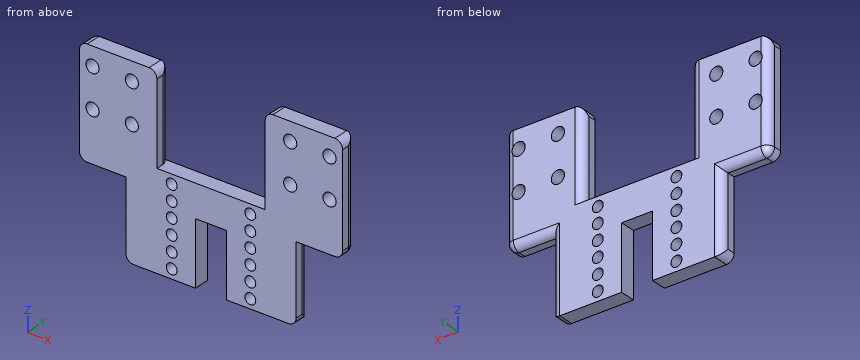
```python
from build123d import *

# Parameters (mm, degrees)
BOSS_EXTRUDE1_DEPTH  = 10
SKETCH2_R            = 4.25
CUT_EXTRUDE1_DEPTH   = 10
SKETCH3_R            = 3.5
CUT_EXTRUDE2_DEPTH   = 10
LPATTERN1_COUNT      = 2
LPATTERN1_PITCH      = 50.8
LPATTERN1_COUNT_DIR2 = 6
LPATTERN1_PITCH_DIR2 = 10
SKETCH4_W            = 30
SKETCH4_H            = 50
CUT_EXTRUDE3_DEPTH   = 10
FILLET1_R            = 5
SKETCH5_W            = 20
SKETCH5_H            = 41
CUT_EXTRUDE4_DEPTH   = 10


with BuildPart() as part:
    # Sketch1 → Boss-Extrude1 (new body)
    with BuildSketch(Plane(origin=(0, 0, 0), x_dir=(1, 0, 0), z_dir=(0, 1, 0))):
        Polygon((0, 0), (50, 0), (120, 0), (170, 0), (170, -119.75), (120, -119.75), (120, -62), (50, -62), (50, -119.75), (0, -119.75), align=None)
    extrude(amount=BOSS_EXTRUDE1_DEPTH)

    # Sketch2 → Cut-Extrude1 (cut)
    with BuildSketch(Plane(origin=(0, 10, 0), x_dir=(1, 0, 0), z_dir=(0, 1, 0))):
        with Locations(Location((33.85, -82.35, 0), (0, 0, 270))):
            Circle(SKETCH2_R)
        with Locations(Location((8.45, -82.35, 0), (0, 0, 270))):
            Circle(SKETCH2_R)
        with Locations(Location((33.85, -107.75, 0), (0, 0, 270))):
            Circle(SKETCH2_R)
        with Locations(Location((8.45, -107.75, 0), (0, 0, 270))):
            Circle(SKETCH2_R)
        with Locations(Location((161.55, -107.75, 0), (0, 0, 270))):
            Circle(SKETCH2_R)
        with Locations(Location((136.15, -107.75, 0), (0, 0, 270))):
            Circle(SKETCH2_R)
        with Locations(Location((136.15, -82.35, 0), (0, 0, 270))):
            Circle(SKETCH2_R)
        with Locations(Location((161.55, -82.35, 0), (0, 0, 270))):
            Circle(SKETCH2_R)
    extrude(amount=-CUT_EXTRUDE1_DEPTH, mode=Mode.SUBTRACT)

    # Sketch3 → Cut-Extrude2 (cut)
    with BuildSketch(Plane(origin=(0, 10, 0), x_dir=(1, 0, 0), z_dir=(0, 1, 0))):
        with Locations(Location((59.6, -6, 0), (0, 0, 270))):
            Circle(SKETCH3_R)
    cut_extrude2 = extrude(amount=-CUT_EXTRUDE2_DEPTH, mode=Mode.SUBTRACT)

    # LPattern1: Cut-Extrude2 2 × 6
    with Locations(*[(i * LPATTERN1_PITCH, 0, j * LPATTERN1_PITCH_DIR2) for i in range(LPATTERN1_COUNT) for j in range(LPATTERN1_COUNT_DIR2) if (i, j) != (0, 0)]):
        add(cut_extrude2, mode=Mode.SUBTRACT)

    # Sketch4 → Cut-Extrude3 (cut)
    with BuildSketch(Plane(origin=(0, 10, 0), x_dir=(1, 0, 0), z_dir=(0, 1, 0))):
        with Locations((15, -25)):
            Rectangle(SKETCH4_W, SKETCH4_H)
        with Locations((155, -25)):
            Rectangle(SKETCH4_W, SKETCH4_H)
    extrude(amount=-CUT_EXTRUDE3_DEPTH, mode=Mode.SUBTRACT)

    # Fillet1
    # the kernel refuses this fillet: 5 mm, written as the material it takes off along each edge
    with BuildSketch(Plane(origin=(5, 5, 55), x_dir=(0, 0, -1), z_dir=(0, 1, 0))) as fillet1_piece_1_section:
        Polygon((0, 0), (FILLET1_R, 0), (FILLET1_R, FILLET1_R), (0, FILLET1_R), align=None)
    fillet1_piece_1 = extrude(amount=FILLET1_R, mode=Mode.PRIVATE)
    fillet1_piece_1 = fillet1_piece_1 - Plane(origin=(5, 5, 55), x_dir=(0.7071067811865476, 0, 0.7071067811865475), z_dir=(0, 1, 0)) * Sphere(FILLET1_R, mode=Mode.PRIVATE)
    add(fillet1_piece_1, mode=Mode.SUBTRACT)
    with BuildSketch(Plane(origin=(165, 5, 55), x_dir=(1, 0, 0), z_dir=(0, 1, 0))) as fillet1_piece_2_section:
        Polygon((0, 0), (FILLET1_R, 0), (FILLET1_R, FILLET1_R), (0, FILLET1_R), align=None)
    fillet1_piece_2 = extrude(amount=FILLET1_R, mode=Mode.PRIVATE)
    fillet1_piece_2 = fillet1_piece_2 - Plane(origin=(165, 5, 55), x_dir=(-0.7071067811865475, 0, 0.7071067811865476), z_dir=(0, 1, 0)) * Sphere(FILLET1_R, mode=Mode.PRIVATE)
    add(fillet1_piece_2, mode=Mode.SUBTRACT)
    with BuildSketch(Plane(origin=(0, 10, 132.25), x_dir=(1, 0, 0), z_dir=(0, 0, -1)), Plane(origin=(170, 10, 55), x_dir=(-1, 0, 0), z_dir=(0, 0, 1))) as fillet1_piece_3:
        with BuildLine():
            CenterArc((FILLET1_R, FILLET1_R), FILLET1_R, 180, 90)
            Line((0, FILLET1_R), (0, 0))
            Line((0, 0), (FILLET1_R, 0))
        make_face()
    extrude(amount=77.25, mode=Mode.SUBTRACT)
    with BuildSketch(Plane(origin=(0, 5, 50), x_dir=(1, 0, 0), z_dir=(0, -1, 0)), Plane(origin=(170, 5, 50), x_dir=(0, 0, 1), z_dir=(0, -1, 0))) as fillet1_piece_4:
        with BuildLine():
            CenterArc((FILLET1_R, FILLET1_R), FILLET1_R, 180, 90)
            Line((0, FILLET1_R), (0, 0))
            Line((0, 0), (FILLET1_R, 0))
        make_face()
    extrude(amount=17.5, mode=Mode.SUBTRACT)
    with BuildSketch(Plane(origin=(30, 22.5, 0), x_dir=(1, 0, 0), z_dir=(0, -1, 0))) as fillet1_piece_5:
        with BuildLine():
            CenterArc((FILLET1_R, FILLET1_R), FILLET1_R, 180, 90)
            Line((0, FILLET1_R), (0, 0))
            Line((0, 0), (FILLET1_R, 0))
        make_face()
    extrude(amount=35, mode=Mode.SUBTRACT)
    with BuildSketch(Plane(origin=(30, 10, 50), x_dir=(0, 0, 1), z_dir=(-1, 0, 0))) as fillet1_piece_6:
        with BuildLine():
            CenterArc((FILLET1_R, -FILLET1_R), FILLET1_R, 90, 90)
            Line((0, -FILLET1_R), (0, 0))
            Line((0, 0), (FILLET1_R, 0))
        make_face()
    extrude(amount=25, mode=Mode.SUBTRACT)
    with BuildSketch(Plane(origin=(30, 10, -12.5), x_dir=(1, 0, 0), z_dir=(0, 0, 1)), Plane(origin=(140, 10, -12.5), x_dir=(0, -1, 0), z_dir=(0, 0, 1))) as fillet1_piece_7:
        with BuildLine():
            CenterArc((FILLET1_R, -FILLET1_R), FILLET1_R, 90, 90)
            Line((0, -FILLET1_R), (0, 0))
            Line((0, 0), (FILLET1_R, 0))
        make_face()
    extrude(amount=62.5, mode=Mode.SUBTRACT)
    with BuildSketch(Plane(origin=(140, 22.5, 0), x_dir=(-1, 0, 0), z_dir=(0, -1, 0)), Plane(origin=(170, -12.5, 119.75), x_dir=(-1, 0, 0), z_dir=(0, 1, 0)), Plane(origin=(120, -12.5, 119.75), x_dir=(0, 0, -1), z_dir=(0, 1, 0)), Plane(origin=(50, -12.5, 119.75), x_dir=(-1, 0, 0), z_dir=(0, 1, 0)), Plane(origin=(0, -12.5, 119.75), x_dir=(0, 0, -1), z_dir=(0, 1, 0))) as fillet1_piece_8:
        with BuildLine():
            CenterArc((FILLET1_R, -FILLET1_R), FILLET1_R, 90, 90)
            Line((0, -FILLET1_R), (0, 0))
            Line((0, 0), (FILLET1_R, 0))
        make_face()
    extrude(amount=35, mode=Mode.SUBTRACT)
    with BuildSketch(Plane(origin=(140, 10, 50), x_dir=(0, 0, 1), z_dir=(1, 0, 0))) as fillet1_piece_9:
        with BuildLine():
            CenterArc((FILLET1_R, FILLET1_R), FILLET1_R, 180, 90)
            Line((0, FILLET1_R), (0, 0))
            Line((0, 0), (FILLET1_R, 0))
        make_face()
    extrude(amount=25, mode=Mode.SUBTRACT)
    with BuildSketch(Plane(origin=(50, 10, 62), x_dir=(-1, 0, 0), z_dir=(0, 0, 1)), Plane(origin=(120, 10, 132.25), x_dir=(1, 0, 0), z_dir=(0, 0, -1))) as fillet1_piece_10:
        with BuildLine():
            CenterArc((FILLET1_R, FILLET1_R), FILLET1_R, 180, 90)
            Line((0, FILLET1_R), (0, 0))
            Line((0, 0), (FILLET1_R, 0))
        make_face()
    extrude(amount=70.25, mode=Mode.SUBTRACT)
    with BuildSketch(Plane(origin=(30, 10, -12.5), x_dir=(1, 0, 0), z_dir=(0, 0, 1))) as fillet1_piece_11a_section:
        with BuildLine():
            CenterArc((FILLET1_R, -FILLET1_R), FILLET1_R, 90, 90)
            Line((0, -FILLET1_R), (0, 0))
            Line((0, 0), (FILLET1_R, 0))
        make_face()
    fillet1_piece_11a = extrude(amount=75, mode=Mode.PRIVATE)
    fillet1_piece_11a = split(fillet1_piece_11a, bisect_by=Plane(origin=(31.131975571, 8.868024429, 50), z_dir=(0, 0, 1)), keep=Keep.TOP, mode=Mode.PRIVATE)
    with BuildSketch(Plane(origin=(42.5, 10, 50), x_dir=(0, 0, 1), z_dir=(-1, 0, 0))) as fillet1_piece_11b_section:
        with BuildLine():
            CenterArc((FILLET1_R, -FILLET1_R), FILLET1_R, 90, 90)
            Line((0, -FILLET1_R), (0, 0))
            Line((0, 0), (FILLET1_R, 0))
        make_face()
    fillet1_piece_11b = extrude(amount=37.5, mode=Mode.PRIVATE)
    fillet1_piece_11b = split(fillet1_piece_11b, bisect_by=Plane(origin=(30, 8.868024429, 51.131975571), z_dir=(1, 0, 0)), keep=Keep.TOP, mode=Mode.PRIVATE)
    fillet1_piece_11 = fillet1_piece_11a & fillet1_piece_11b
    add(fillet1_piece_11, mode=Mode.SUBTRACT)
    with BuildSketch(Plane(origin=(140, 10, -12.5), x_dir=(0, -1, 0), z_dir=(0, 0, 1))) as fillet1_piece_12a_section:
        with BuildLine():
            CenterArc((FILLET1_R, -FILLET1_R), FILLET1_R, 90, 90)
            Line((0, -FILLET1_R), (0, 0))
            Line((0, 0), (FILLET1_R, 0))
        make_face()
    fillet1_piece_12a = extrude(amount=75, mode=Mode.PRIVATE)
    fillet1_piece_12a = split(fillet1_piece_12a, bisect_by=Plane(origin=(138.868024429, 8.868024429, 50), z_dir=(0, 0, 1)), keep=Keep.TOP, mode=Mode.PRIVATE)
    with BuildSketch(Plane(origin=(127.5, 10, 50), x_dir=(0, 0, 1), z_dir=(1, 0, 0))) as fillet1_piece_12b_section:
        with BuildLine():
            CenterArc((FILLET1_R, FILLET1_R), FILLET1_R, 180, 90)
            Line((0, FILLET1_R), (0, 0))
            Line((0, 0), (FILLET1_R, 0))
        make_face()
    fillet1_piece_12b = extrude(amount=37.5, mode=Mode.PRIVATE)
    fillet1_piece_12b = split(fillet1_piece_12b, bisect_by=Plane(origin=(140, 8.868024429, 51.131975571), z_dir=(-1, 0, 0)), keep=Keep.TOP, mode=Mode.PRIVATE)
    fillet1_piece_12 = fillet1_piece_12a & fillet1_piece_12b
    add(fillet1_piece_12, mode=Mode.SUBTRACT)

    # Sketch5 → Cut-Extrude4 (cut)
    with BuildSketch(Plane(origin=(0, 10, 0), x_dir=(1, 0, 0), z_dir=(0, 1, 0))):
        with Locations((85, -20.5)):
            Rectangle(SKETCH5_W, SKETCH5_H)
    extrude(amount=-CUT_EXTRUDE4_DEPTH, mode=Mode.SUBTRACT)


solid = part.part
```
For this review, take the finished solid that the model builds, in its own axes (mm). Coordinates: 2 decimals unless noted, no trailing zeros. Loops run counter-clockwise (first coordinate to the right, second up) from the corner with the lowest first, then second, coordinate; pieces in that order, holes last. Notation, with made-up numbers: (-2.75, -21.5) -> (4.25, -21.5) arc R28 cw to (4.25, 9.5) -> close; hole circle Ø3 at (67, 65). An arc over 180 degrees is marked (long way). Return JSON: item names as keys, results as strings. Group by question number.
(1) To check wall thickness, follow L1, parallel to X at y = 5.25, z = 107.75; L2, parallel to Z at x = 8.45, y = 5; L3, parallel to X at y = 4, z = 16. State the ranges of each line that lie inside material, in increasing order.
(2) For pin 1 Ø4 at (x, z) = (110.4, 6) entering from -Y; pin 2 Ø2.5 at (y, z) = (1.5, 18) entering from -X; pin 3 Ø2 at (x, z) = (138.5, 98.5) entering from -Y; pin 4 Ø1.5 at (x, y) = (18.5, 2.5) entering from -Z, all flat-tipped, find the tip position at first contact; note any pin that passes through.
(3) Consider section B-B, the plane x = 8.45. Give the boundary of the cut face in (y, z), plus the area to 3 significant figures.
(4) Consider section D-D, the plane x = 110.4. Give the boundary of the cut face in (y, z).
(5) Consider section C-C, the plane z = 65. Give the boundary of the cut face in (x, y), plus the area to 3 significant figures.
(6) Consider section A-A, the plane z = 46. Give the boundary of the cut face in (x, y), plus the area to 3 significant figures.
Results below:
{
 "1": {"L1": "x = 0.01 to 4.2, 12.7 to 29.6, 38.1 to 49.99, 120.01 to 131.9, 140.4 to 157.3, 165.8 to 169.99", "L2": "z = 50 to 78.1, 86.6 to 103.5, 112 to 119.75", "L3": "x = 30 to 56.1, 63.1 to 75, 95 to 106.9, 113.9 to 140"},
 "2": {"pin 1": "passes through", "pin 2": "stops at x = 30", "pin 3": "stops at y = 0", "pin 4": "stops at z = 50"},
 "3": {"outline": "(0, 50) -> (5, 50) arc R5 ccw to (10, 55) -> (10, 78.1) -> (0, 78.1) -> close; (0, 86.6) -> (10, 86.6) -> (10, 103.5) -> (0, 103.5) -> close; (0, 112) -> (10, 112) -> (10, 119.75) -> (0, 119.75) -> close", "area": "522 mm2"},
 "4": {"outline": "(0, 0) -> (10, 0) -> (10, 2.5) -> (0, 2.5) -> close; (0, 9.5) -> (10, 9.5) -> (10, 12.5) -> (0, 12.5) -> close; (0, 19.5) -> (10, 19.5) -> (10, 22.5) -> (0, 22.5) -> close; (0, 29.5) -> (10, 29.5) -> (10, 32.5) -> (0, 32.5) -> close; (0, 39.5) -> (10, 39.5) -> (10, 42.5) -> (0, 42.5) -> close; (0, 49.5) -> (10, 49.5) -> (10, 52.5) -> (0, 52.5) -> close; (0, 59.5) -> (10, 59.5) -> (10, 62) -> (0, 62) -> close"},
 "5": {"outline": "(0, 0) -> (50, 0) -> (50, 5) arc R5 ccw to (45, 10) -> (5, 10) arc R5 ccw to (0, 5) -> close; (120, 0) -> (170, 0) -> (170, 5) arc R5 ccw to (165, 10) -> (125, 10) arc R5 ccw to (120, 5) -> close", "area": "979 mm2"},
 "6": {"outline": "(30, 0) -> (56.1, 0) -> (56.1, 10) -> (35, 10) arc R5 ccw to (30, 5) -> close; (63.1, 0) -> (106.9, 0) -> (106.9, 10) -> (63.1, 10) -> close; (113.9, 0) -> (140, 0) -> (140, 5) arc R5 ccw to (135, 10) -> (113.9, 10) -> close", "area": "949 mm2"}
}
